from build123d import *

# Parameters (mm, degrees)
SKETCH1_W           = 26
SKETCH1_H           = 17
BOSS_EXTRUDE1_DEPTH = 4
SKETCH2_W           = 3
SKETCH2_H           = 17
BOSS_EXTRUDE2_DEPTH = 37
SKETCH3_R           = 2.75
CUT_EXTRUDE1_DEPTH  = 47.013584951
FILLET1_R           = 3
FILLET2_R           = 5
SKETCH5_R           = 7
BOSS_EXTRUDE3_DEPTH = 2
CUT_EXTRUDE3_REACH  = 45.843
SKETCH7_R           = 2.25
CUT_EXTRUDE4_DEPTH  = 4
CHAMFER1_SIZE       = 2


with BuildPart() as part:
    # Sketch1 → Boss-Extrude1 (new body)
    with BuildSketch(Plane(origin=(0, 0, 0), x_dir=(0, 0, -1), z_dir=(1, 0, 0))):
        Rectangle(SKETCH1_W, SKETCH1_H)
    extrude(amount=BOSS_EXTRUDE1_DEPTH)

    # Sketch2 → Boss-Extrude2 (add)
    with BuildSketch(Plane.ZY):
        with Locations((-11.5, 0)):
            Rectangle(SKETCH2_W, SKETCH2_H)
        with Locations((11.5, 0)):
            Rectangle(SKETCH2_W, SKETCH2_H)
    extrude(amount=BOSS_EXTRUDE2_DEPTH)

    # Sketch3 → Cut-Extrude1 (cut, through all)
    with BuildSketch(Plane.XY.offset(13)):
        with Locations((-29.5, 0)):
            Circle(SKETCH3_R)
    extrude(amount=-CUT_EXTRUDE1_DEPTH, mode=Mode.SUBTRACT)

    # Fillet1
    fillet1_edges = [part.edges().sort_by_distance(p)[0] for p in [
        (4, 0, 13),
        (0, 0, -10),
        (0, 0, 10),
        (4, 0, -13),
    ]]
    fillet(fillet1_edges, radius=FILLET1_R)

    # Fillet2
    fillet2_edges = [part.edges().sort_by_distance(p)[0] for p in [
        (-37, -8.5, -11.5),
        (-37, 8.5, -11.5),
        (-37, 8.5, 11.5),
        (-37, -8.5, 11.5),
    ]]
    fillet(fillet2_edges, radius=FILLET2_R)

    # Sketch5 → Boss-Extrude3 (add)
    with BuildSketch(Plane.ZY):
        Circle(SKETCH5_R)
    extrude(amount=BOSS_EXTRUDE3_DEPTH)

    # Sketch7 → Cut-Extrude3 (cut, up to next)
    with BuildSketch(Plane(origin=(4, 0, 0), x_dir=(0, 0, -1), z_dir=(1, 0, 0)), mode=Mode.PRIVATE) as cut_extrude3_sk1:
        Circle(SKETCH7_R)
    cut_extrude3_tool1 = extrude(cut_extrude3_sk1.sketch, amount=-CUT_EXTRUDE3_REACH, mode=Mode.PRIVATE) & part.part
    add(cut_extrude3_tool1.solids().sort_by_distance((4, 0, 0))[0], mode=Mode.SUBTRACT)

    # Sketch8 → Cut-Extrude4 (cut)
    with BuildSketch(Plane.ZY.offset(2)):
        Polygon((0, 4.330127019), (-3.75, 2.165063509), (-3.75, -2.165063509), (0, -4.330127019), (3.75, -2.165063509), (3.75, 2.165063509), align=None)
    extrude(amount=-CUT_EXTRUDE4_DEPTH, mode=Mode.SUBTRACT)

    # Chamfer1
    # the kernel refuses this chamfer: 2 mm, written as the material it adds along each edge
    with BuildSketch(Plane(origin=(0, 0, 0), x_dir=(0, 0, 1), z_dir=(0, -1, 0))) as chamfer1_piece_1_section:
        Polygon((7 + CHAMFER1_SIZE, 0), (7, CHAMFER1_SIZE), (7, 0), align=None)
    chamfer1_piece_1 = revolve(axis=Axis((0, 0, 0), (-1, 0, 0)), revolution_arc=180, mode=Mode.PRIVATE)
    chamfer1_piece_1 = split(chamfer1_piece_1, bisect_by=Plane(origin=(-0.945270908, 8.5, 0), z_dir=(0, -1, 0)), keep=Keep.TOP, mode=Mode.PRIVATE)
    chamfer1_piece_1 = split(chamfer1_piece_1, bisect_by=Plane(origin=(-2, 8.001839451, 0), z_dir=(1, 0, 0)), keep=Keep.TOP, mode=Mode.PRIVATE)
    add(chamfer1_piece_1)
    with BuildSketch(Plane(origin=(0, 0, 0), x_dir=(0, 0, -1), z_dir=(0, 1, 0))) as chamfer1_piece_2_section:
        Polygon((7 + CHAMFER1_SIZE, 0), (7, CHAMFER1_SIZE), (7, 0), align=None)
    chamfer1_piece_2 = revolve(axis=Axis((0, 0, 0), (-1, 0, 0)), revolution_arc=180, mode=Mode.PRIVATE)
    chamfer1_piece_2 = split(chamfer1_piece_2, bisect_by=Plane(origin=(-0.945270905, -8.5, 0), z_dir=(0, 1, 0)), keep=Keep.TOP, mode=Mode.PRIVATE)
    chamfer1_piece_2 = split(chamfer1_piece_2, bisect_by=Plane(origin=(-2, -8.001839447, 0), z_dir=(1, 0, 0)), keep=Keep.TOP, mode=Mode.PRIVATE)
    add(chamfer1_piece_2)


solid = part.part
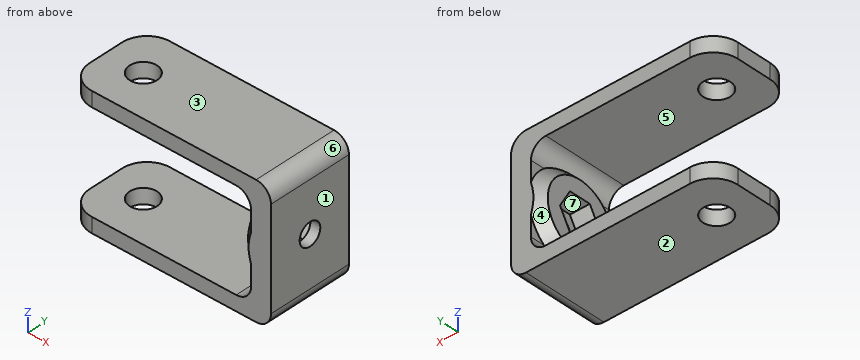
Design review of the part built by this model. Coordinates are the model's own, in mm. Face numbers are marked on the shaded views. A direction names the side the tool comes from. Round coordinates to 2 decimals unless told otherwise and drop trailing zeros. Write each loop counter-clockwise with the first axis right and the second up, starting at its lowest first coordinate (ties: lowest second). Pieces come first, ordered by that corner, then holes. Notation, with made-up numbers: (-14, 28) - (25, 28) arc R5 cw to (25, 37) - close; hole circle Ø9 at (30, 13.5). An arc over 180 degrees is marked (long way). Use a Markdown table: item, result. Add a question column.
1. We need section A-A (x = -14). State the section outline as (y, z) points, then the cut area to 3 significant figures.
2. Clearance check with flat-ended pins moving along their axes: pin 1 (1.4 mm diameter, centred on y = 6.5, z = -5, fed in from -X); pin 2 (0.9 mm diameter, centred on y = -7.5, z = -5, fed in from -X); pin 3 (6 mm diameter, centred on y = -1, z = 1.5, fed in from -X). State where each tip first meets the part, or that it passes through.
3. We need section C-C (y = 0). Count the separate pieces of the cut face and the enclosed holes in it, then the cut area to 3 significant figures.
4. Wall thickness on probe 1 along Y at (x, z) = (-29.5, -10.9); probe 2 along Y at (x, z) = (3.6, 0); probe 3 along Z at (x, y) = (-7, -2): over which ranges is each line inside the solid? List them lowest first.
5. Mouldability with a two-part tool opening along Z and no side actions: class the marked faces 1, 2, 3 and 4 as +Z half, -Z half, draft (parallel to the pull), parting line (faces both ways), or undercut.
6. We need section B-B (x = -29.5). State the section outline as (y, z) points, then the cut area to 3 significant figures.
7. For the marked faces 5, 6 and 7, list the 3-axis set-ups (+Z, -Z, +X, -X, +Y, -Y) from which the entire face can be reached by the end or side of a thin tool; tool diameter is ignored.
Output:
| question | item | result |
|---|---|---|
| 1 | outline | (-8.5, -13) - (8.5, -13) - (8.5, -10) - (-8.5, -10) - close; (-8.5, 10) - (8.5, 10) - (8.5, 13) - (-8.5, 13) - close |
| 1 | area | 102 mm2 |
| 2 | pin 1 | stops at x = -1.5 |
| 2 | pin 2 | stops at x = -0.44 |
| 2 | pin 3 | stops at x = -2 |
| 3 | separate pieces | 4 |
| 3 | enclosed holes | 0 |
| 3 | area | 285 mm2 |
| 4 | probe 1 | y = -8.5 to -2.75, 2.75 to 8.5 |
| 4 | probe 2 | y = -8.5 to -2.25, 2.25 to 8.5 |
| 4 | probe 3 | z = -13 to -10, 10 to 13 |
| 5 | face 1 | draft |
| 5 | face 2 | -Z half |
| 5 | face 3 | +Z half |
| 5 | face 4 | undercut |
| 6 | outline | (-8.5, -13) - (-2.75, -13) - (-2.75, -10) - (-8.5, -10) - close; (-8.5, 10) - (-2.75, 10) - (-2.75, 13) - (-8.5, 13) - close; (2.75, -13) - (8.5, -13) - (8.5, -10) - (2.75, -10) - close; (2.75, 10) - (8.5, 10) - (8.5, 13) - (2.75, 13) - close |
| 6 | area | 69.0 mm2 |
| 7 | face 5 | -X, +Y, -Y |
| 7 | face 6 | +Z, +X, +Y, -Y |
| 7 | face 7 | -X |
